Autodesk Inventor part; units mm, degrees
ref_plane "YZ Plane" through (0, 0, 0) normal (1, 0, 0) x (0, 1, 0)
ref_plane "XZ Plane" through (0, 0, 0) normal (0, 1, 0) x (-1, 0, 0)
ref_plane "XY Plane" through (0, 0, 0) normal (0, 0, 1) x (1, 0, 0)
sketch "Sketch1" plane through (0, 0, 0) normal (0, 1, 0) x (-1, 0, 0)
  line L0 (0, 0) -> (-58, 0)
  line L1 (-58, 0) -> (-58, 5)
  line L2 (-58, 5) -> (0, 5)
  line L3 (0, 5) -> (0, 0)
  line L4 (0, 5) -> (-5, 5)
  line L5 (-5, 5) -> (-5, 47)
  line L6 (-5, 47) -> (0, 47)
  line L7 (0, 47) -> (0, 5)
  line L8 (-58, 5) -> (-53, 5)
  line L9 (-53, 5) -> (-53, 47)
  line L10 (-53, 47) -> (-58, 47)
  line L11 (-58, 47) -> (-58, 5)
  dimension "d0" = 58
  dimension "d1" = 5
  dimension "d2" = 5
  dimension "d3" = 42
  dimension "d4" = 5
  dimension "d5" = 42
extrude "Extrusion1" add sketch "Sketch1" against normal blind 62
sketch "Sketch2" plane through (58, 0, 47) normal (1, 0, 0) x (0, 0, -1)
  line L0 (0, 0) -> (0, -62)
  line L1 (47, -62) -> (0, -62)
  circle A0 centre (21, -12) radius 3
  point P0 (47, 0)
  point P1 (23.5, -62)
  dimension "d8" = 21
  dimension "d9" = 50
  dimension "d10" = 6
sketch "Sketch3" plane through (0, -62, 0) normal (0, -1, 0) x (1, 0, 0)
  line L0 (53, 47) -> (58, 47)
  line L1 (58, 47) -> (63, 47)
  line L2 (63, 47) -> (63, 0)
  line L3 (63, 0) -> (58, 0)
  line L4 (58, 0) -> (58, 47)
  line L5 (0, 0) -> (0, 47)
  line L6 (0, 47) -> (-5, 47)
  line L7 (-5, 47) -> (-5, 0)
  line L8 (-5, 0) -> (0, 0)
  line L9 (0, 0) -> (0, 47)
  line L10 (63, 0) -> (-5, 0)
  line L11 (-5, 0) -> (-5, -5)
  line L12 (-5, -5) -> (63, -5)
  line L13 (63, -5) -> (63, 0)
  dimension "d13" = 5
  dimension "d14" = 5
  dimension "d15" = 5
extrude "Extrusion3" add sketch "Sketch3" against normal blind 8
sketch "Sketch4" plane through (0, -62, 0) normal (0, -1, 0) x (1, 0, 0)
  line L0 (58, 47) -> (58, 0)
  line L1 (63, 47) -> (53, 47)
  line L2 (0, 0) -> (0, 47)
  line L3 (5, 47) -> (-5, 47)
  circle A0 centre (58, 37) radius 2.5
  circle A1 centre (0, 37) radius 2.5
  line L4 (58, 0) -> (0, 0)
  circle A2 centre (16.5, 0) radius 2.5
  circle A3 centre (41.5, 0) radius 2.5
  point P0 (29, 0)
  dimension "d18" = 10
  dimension "d19" = 10
  dimension "d20" = 5
  dimension "d21" = 5
  dimension "d29" = 5
  dimension "d30" = 5
sketch "Sketch5" plane through (0, 0, 0) normal (-1, 0, 0) x (0, 0, 1)
  circle A0 centre (26, -12) radius 3
  circle A1 centre (26, -12) radius 3
  point P0 (0, 0)
extrude "Extrusion5" cut sketch "Sketch5" against normal blind 5
extrude "Extrusion6" cut sketch "Sketch4" against normal blind 5
equation "\"d4\" = d2"
equation "\"d5\" = d3"
equation "\"d14\" = d13"
equation "\"d15\" = d13"
equation "\"d21\" = d20"
equation "\"d29\" = d20"
equation "\"d30\" = d20"
properties part number "top cam mount v02"
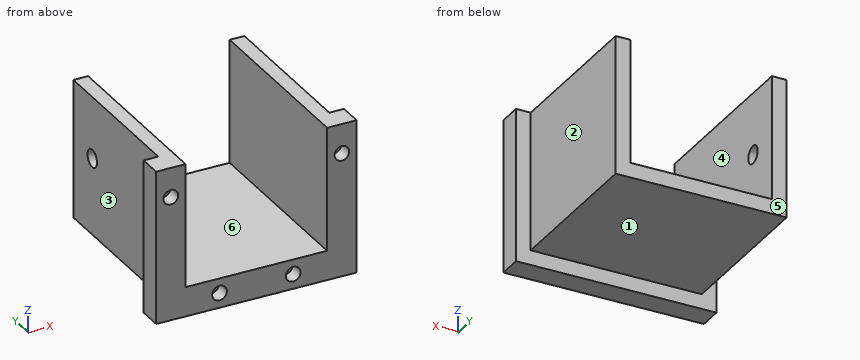
The model under review builds one solid part; all positions refer to its coordinate system, in mm. Face numbers are marked on the shaded views. A direction names the side the tool comes from. Coordinates: 2 decimals unless noted, no trailing zeros. Loops run counter-clockwise (first coordinate to the right, second up) from the corner with the lowest first, then second, coordinate; pieces in that order, holes last. Notation, with made-up numbers: M 86,6 L 132,6 A18 ccw 132,37 Z; hole C 42.25,-3 d9. An arc over 180 degrees is marked long. Put each result on its own line as item: value. Start each with the question number.
Q1. The part is to be moulded in two halves that separate along X. For the marked faces 1, 2, 3 and 4, say which applies: +X half, -X half, draft (parallel to the pull), parting line (faces both ways), or undercut.
Q2. Add section D-D (x = 41.5). Write out the cut boundary in (y, z).
Q3. Add section A-A (z = 37). Write out the cut boundary in (x, y).
Q4. For the marked faces 5 and 6, list the 3-axis set-ups (+Z, -Z, +X, -X, +Y, -Y) from which the entire face can be reached by the end or side of a thin tool; tool diameter is ignored.
Q5. Add section C-C (y = -12). Write out the cut boundary in (x, z), and give its area (3 significant figures).
Q6. Wall thickness on line 1 (X direction, y = -60, z = 37); line 2 (X direction, y = -58, z = 0); line 3 (Z direction, x = 0, y = -59): over which ranges is each line inside the solid? List them lowest first.
Q7. Clearance check with flat-ended pins moving along their axes: pin 1 (23.5 mm diameter, centred on y = -39.5, z = 14, fed in from +X); pin 2 (2 mm diameter, centred on x = 23.5, y = -31.5, fed in from -Z); pin 3 (14 mm diameter, centred on y = -31, z = 14, fed in from -X). State where each tip first meets the part, or that it passes through.
Q8. Add section B-B (z = 26). Write out the cut boundary in (x, y).
Answers:
1. face 1: draft
1. face 2: +X half
1. face 3: -X half
1. face 4: undercut
2. outline: M -62,-5 L -54,-5 L -54,0 L 0,0 L 0,5 L -62,5 L -62,2.5 L -57,2.5 L -57,-2.5 L -62,-2.5 Z
3. outline: M -5,-62 L -2.5,-62 L -2.5,-57 L 2.5,-57 L 2.5,-62 L 5,-62 L 5,0 L 0,0 L 0,-54 L -5,-54 Z; M 53,-62 L 55.5,-62 L 55.5,-57 L 60.5,-57 L 60.5,-62 L 63,-62 L 63,-54 L 58,-54 L 58,0 L 53,0 Z
4. face 5: +Z, -Z, +X, -X, +Y
4. face 6: +Z, +Y, -Y
5. outline: M 0,0 L 58,0 L 58,47 L 53,47 L 53,5 L 5,5 L 5,23 L 0,23 Z; M 0,29 L 5,29 L 5,47 L 0,47 Z
5. area: 680 mm^2
6. line 1: x = -5 to -2.5, 2.5 to 5, 53 to 55.5, 60.5 to 63
6. line 2: x = -5 to 14, 19 to 39, 44 to 63
6. line 3: z = -5 to 34.5, 39.5 to 47
7. pin 1: stops at x = 58
7. pin 2: stops at z = 0
7. pin 3: stops at x = 0
8. outline: M -5,-62 L 5,-62 L 5,-15 L 0,-15 L 0,-54 L -5,-54 Z; M 0,-9 L 5,-9 L 5,0 L 0,0 Z; M 53,-62 L 63,-62 L 63,-54 L 58,-54 L 58,0 L 53,0 Z
